The listing builds one solid part. Answer for the finished solid, in the listing's coordinates (mm). Face numbers are marked on the shaded views. A direction names the side the tool comes from. Give positions to 0.01 mm unless a question says otherwise; leave off trailing zeros. Loops run counter-clockwise (first coordinate to the right, second up) from the corner with the lowest first, then second, coordinate; pieces in that order, holes last. Notation, with made-up numbers: (86, 61.25) - (134, 61.25) arc R16 cw to (134, 77.25) - close; hole circle Ø7 at (34, 86). An arc over 180 degrees is marked (long way). Write item = value, one per line. Start each with the question number.
1) The part is cut by section C-C on z = 21.25. Write down the section's boundary in (x, y), plus the area to 3 significant figures.
2) Which of the six approach directions +Z, -Z, +X, -X, +Y, -Y give full straight-line access (tool end or side, diameter ignored) to the marked faces 1 and 2?
3) The part is cut by section A-A on z = 10.5. Write down the section's boundary in (x, y) (3 decimals), plus the area to 3 significant figures.
4) Consider probe 1 along Y at (x, z) = (166, 19); probe 2 along X at (y, z) = (43.5, 22); probe 3 along Z at (x, y) = (128, 26). Determine where each line is inside the solid, lowest interval first.
5) The part is cut by section D-D on y = 54. Write down the section's boundary in (x, z).
6) The mould has two halves that part along Y. Classify the marked faces 3, 4, 5 and 6: +Y half, -Y half, draft (parallel to the pull), parting line (faces both ways), or undercut.
7) The part is cut by section B-B on x = 69.5. Write down the section's boundary in (y, z), plus the area to 3 significant figures.
8) Flat-ended cylindrical pins translate along their axes: P1, Ø10, axis at x = 55.5, y = 20, coming from the +Z side; P2, Ø7, axis at x = 44.5, y = 88, coming from the +Z side; P3, Ø4, axis at x = 25.5, y = 90, coming from the -Z side; P4, Ø4, axis at y = 84, z = 4, coming from the +X side. Find the tip coordinate at first contact, or state that the pin passes through.
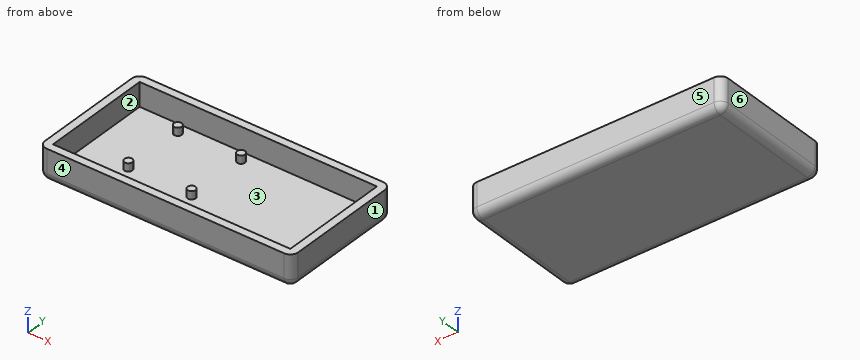
from build123d import *

# Parameters (mm, degrees)
F0_W     = 203.2
F0_H     = 101.6
F1_DEPTH = 25.4
F2_R     = 6.35
F3_T     = 6.35
F5_DEPTH = 6.35


# Not quite as in the source:
# - a shell that OpenCascade refuses in one call is made with other operations: the cavity is built on its own and cut out


with BuildPart() as f1:
    # F0 (on Top) → F1 (new body)
    with BuildSketch(Plane.XY):
        with Locations((101.6, 50.8)):
            Rectangle(F0_W, F0_H)
    extrude(amount=F1_DEPTH)

    # F2
    f2_edges = [f1.edges().sort_by_distance(p)[0] for p in [
        (0, 0, 12.7),
        (203.2, 0, 12.7),
        (0, 101.6, 12.7),
        (203.2, 101.6, 12.7),
        (101.6, 101.6, 0),
        (0, 50.8, 0),
        (101.6, 0, 0),
        (203.2, 50.8, 0),
    ]]
    fillet(f2_edges, radius=F2_R)

    # F3: shell of thickness 6.35, made by hand


with BuildPart() as f3_core1:
    # F3_t2: copy of F1
    add(f1.part)

    # the walls: a layer under each face that stays
    f3_faces = [f3_core1.faces().sort_by_distance(p)[0] for p in [
        (0, 50.8, 15.875),
        (101.6, 101.6, 15.875),
        (101.6, 0, 15.875),
        (203.2, 50.8, 15.875),
        (101.6, 50.8, 0),
    ]]
    thicken(f3_faces, amount=-F3_T, mode=Mode.SUBTRACT)


with BuildPart() as f1_1:
    add(f1.part)

    # what is left inside the walls is the cavity
    f3_cavity = [f3_core1.part.solids().sort_by_distance(p)[0] for p in [
        (101.6, 35.983333, 25.3365),
    ]]
    add(f3_cavity, mode=Mode.SUBTRACT)

    # F4 (on face) → F5 (join)
    with BuildSketch(Plane.XY.offset(6.35)):
        with BuildLine():
            Line((43.5933910498, 86.815246595), (46.7683910498, 86.815246595))
            ThreePointArc((46.7683910498, 86.815246595), (41.3483270196, 89.0603106253), (43.5933910498, 83.640246595))
            Line((43.5933910498, 83.640246595), (43.5933910498, 86.815246595))
        make_face()
        with BuildLine():
            ThreePointArc((43.5933910498, 83.640246595), (45.8384550801, 84.5701825647), (46.7683910498, 86.815246595))
            Line((46.7683910498, 86.815246595), (43.5933910498, 86.815246595))
            Line((43.5933910498, 86.815246595), (43.5933910498, 83.640246595))
        make_face()
        with BuildLine():
            ThreePointArc((97.5683910498, 86.815246595), (94.3933910498, 89.990246595), (91.2183910498, 86.815246595))
            Line((91.2183910498, 86.815246595), (94.3933910498, 86.815246595))
            Line((94.3933910498, 86.815246595), (94.3933910498, 83.640246595))
            ThreePointArc((94.3933910498, 83.640246595), (96.6384550801, 84.5701825647), (97.5683910498, 86.815246595))
        make_face()
        with BuildLine():
            Line((94.3933910498, 86.815246595), (91.2183910498, 86.815246595))
            ThreePointArc((91.2183910498, 86.815246595), (92.1483270196, 84.5701825647), (94.3933910498, 83.640246595))
            Line((94.3933910498, 83.640246595), (94.3933910498, 86.815246595))
        make_face()
        with BuildLine():
            Line((94.3933910498, 36.015246595), (94.3933910498, 39.190246595))
            ThreePointArc((94.3933910498, 39.190246595), (92.1483270196, 38.2603106253), (91.2183910498, 36.015246595))
            Line((91.2183910498, 36.015246595), (94.3933910498, 36.015246595))
        make_face()
        with BuildLine():
            ThreePointArc((46.7683910498, 36.015246595), (45.8384550801, 38.2603106253), (43.5933910498, 39.190246595))
            Line((43.5933910498, 39.190246595), (43.5933910498, 36.015246595))
            Line((43.5933910498, 36.015246595), (46.7683910498, 36.015246595))
        make_face()
        with BuildLine():
            Line((43.5933910498, 36.015246595), (43.5933910498, 39.190246595))
            ThreePointArc((43.5933910498, 39.190246595), (41.3483270196, 33.7701825647), (46.7683910498, 36.015246595))
            Line((46.7683910498, 36.015246595), (43.5933910498, 36.015246595))
        make_face()
        with BuildLine():
            ThreePointArc((97.5683910498, 36.015246595), (96.6384550801, 38.2603106253), (94.3933910498, 39.190246595))
            Line((94.3933910498, 39.190246595), (94.3933910498, 36.015246595))
            Line((94.3933910498, 36.015246595), (91.2183910498, 36.015246595))
            ThreePointArc((91.2183910498, 36.015246595), (94.3933910498, 32.840246595), (97.5683910498, 36.015246595))
        make_face()
    extrude(amount=F5_DEPTH)


solid = f1_1.part
Answer below:
q1.outline = (0, 6.35) arc R6.35 ccw to (6.35, 0) - (196.85, 0) arc R6.35 ccw to (203.2, 6.35) - (203.2, 95.25) arc R6.35 ccw to (196.85, 101.6) - (6.35, 101.6) arc R6.35 ccw to (0, 95.25) - close; hole (6.35, 6.35) - (196.85, 6.35) - (196.85, 95.25) - (6.35, 95.25) - close
q1.area = 3,680 mm2
q2.face_1 = +Z, -Z, +X, +Y, -Y
q2.face_2 = +Z
q3.outline = (0, 6.35) arc R6.35 ccw to (6.35, 0) - (196.85, 0) arc R6.35 ccw to (203.2, 6.35) - (203.2, 95.25) arc R6.35 ccw to (196.85, 101.6) - (6.35, 101.6) arc R6.35 ccw to (0, 95.25) - close; circle Ø6.35 at (43.593, 36.015); circle Ø6.35 at (43.593, 86.815); circle Ø6.35 at (94.393, 36.015); circle Ø6.35 at (94.393, 86.815); hole (6.35, 6.35) - (196.85, 6.35) - (196.85, 95.25) - (6.35, 95.25) - close
q3.area = 3,800 mm2
q4.probe_1 = 0 to 6.35, 95.25 to 101.6
q4.probe_2 = 0 to 6.35, 196.85 to 203.2
q4.probe_3 = 0 to 6.35
q5.outline = (0, 6.35) arc R6.35 ccw to (6.35, 0) - (196.85, 0) arc R6.35 ccw to (203.2, 6.35) - (203.2, 25.4) - (196.85, 25.4) - (196.85, 6.35) - (6.35, 6.35) - (6.35, 25.4) - (0, 25.4) - close
q6.face_3 = undercut
q6.face_4 = -Y half
q6.face_5 = +Y half
q6.face_6 = draft
q7.outline = (0, 6.35) arc R6.35 ccw to (6.35, 0) - (95.25, 0) arc R6.35 ccw to (101.6, 6.35) - (101.6, 25.4) - (95.25, 25.4) - (95.25, 6.35) - (6.35, 6.35) - (6.35, 25.4) - (0, 25.4) - close
q7.area = 870 mm2
q8.P1 = 6.35
q8.P2 = 12.7
q8.P3 = 0
q8.P4 = 203.19
